Here's how the part is built. I have some questions about the finished solid (model axes, mm). A direction names the side the tool comes from. Give positions to 0.01 mm unless a question says otherwise; leave off trailing zeros. Write each loop counter-clockwise with the first axis right and the second up, starting at its lowest first coordinate (ties: lowest second). Pieces come first, ordered by that corner, then holes. Notation, with made-up numbers: (81, 73.5) - (94, 73.5) arc R20 ccw to (94, 111.5) - close; hole circle Ø3 at (38, -20.5). An arc over 180 degrees is marked (long way). One line per item, written item: value. Start each with the question number.
1) Imagine slicing it at B-B on x = 10. Write out the boundary of the cut face in (y, z), plus the area to 3 significant figures.
2) On a 3-axis mill with a long thin cutter (end or side, diameter ignored), from which of +Z, -Z, +X, -X, +Y, -Y can I reach the whole of each face in a straight line? I mean faces 3 (the flat face through (0, 15, 216)), 4 (the flat face through (22.7, -3, 215.9)), 5 (the flat face through (10, -2, 268)), 6 (the flat face through (10, -5, 274)). Say none if no direction works.
3) I'm going to push flat-ended pins straight in: P1, Ø2, axis at x = 0.5, y = 3.5, coming from the +Z side; P2, Ø0.6, axis at x = 13, y = -1, coming from the +Z side; P3, Ø1.2, axis at y = -5, z = 202, coming from the +X side; P4, Ø5, axis at y = 7, z = 186, coming from the +X side. Where does each tip first touch, or does it pass through?
4) Imagine slicing it at A-A on z = 215. Write out the boundary of the cut face in (x, y).
5) We'd pull the mould along Z, two halves only. Please class faces 1 (the flat face through (-2, -1, 216)), 2 (the cylindrical face through (10.35, -2.58, 158.44)): +Z half, -Z half, draft (parallel to the pull), parting line (faces both ways), or undercut.
6) Please list where these lines run through material, in increasing order: L1, parallel to Z at x = 10, y = -4; L2, parallel to Y at x = -1, z = 160; L3, parallel to Y at x = -4, z = 262. Write a range as [from, to].
7) Imagine slicing it at D-D on z = 252. Write out the boundary of the cut face in (x, y), plus the area to 3 significant figures.
from build123d import *

# Parameters (mm, degrees)
BOSS_EXTRUDE1_DEPTH            = 130
FILLET1_R                      = 1.5
SKETCH2_W                      = 130
SKETCH2_H                      = 3
BOSS_EXTRUDE2_DEPTH            = 10
SKETCH4_W                      = 13
SKETCH4_H                      = 130
BOSS_EXTRUDE3_DEPTH            = 4
SKETCH6_W                      = 3
SKETCH6_H                      = 130
BOSS_EXTRUDE4_DEPTH            = 10
SKETCH5_W                      = 130
SKETCH5_H                      = 13
BOSS_EXTRUDE5_DEPTH            = 4
CSK_FOR_M3_SFHCS1_D            = 3.2
CSK_FOR_M3_SFHCS1_CSINK_D      = 6.72
CSK_FOR_M3_SFHCS1_CSINK_ANGLE  = 90
CSK_FOR_M3_SFHCS2_D            = 3.2
CSK_FOR_M3_SFHCS2_CSINK_D      = 6.72
CSK_FOR_M3_SFHCS2_CSINK_ANGLE  = 90
SKETCH13_W                     = 12
SKETCH13_H                     = 24
CUT_EXTRUDE1_DEPTH             = 2
F_4_4_4_4_DIAMETER_HOLE1_D     = 4.4
F_4_4_4_4_DIAMETER_HOLE1_DEPTH = 3
SKETCH16_W                     = 24
SKETCH16_H                     = 12
CUT_EXTRUDE2_DEPTH             = 2
F_4_4_4_4_DIAMETER_HOLE2_D     = 4.4
F_4_4_4_4_DIAMETER_HOLE2_DEPTH = 3
F_4_4_4_4_DIAMETER_HOLE3_D     = 4.4
F_4_4_4_4_DIAMETER_HOLE4_D     = 4.4


with BuildPart() as part:
    # Sketch1 → Boss-Extrude1 (new body)
    with BuildSketch(Plane.XY.offset(280)):
        Polygon((-7, 4), (4, -7), (7, -7), (7, -3), (20, -3), (20, 0), (0, 0), (0, 20), (-3, 20), (-3, 7), (-7, 7), align=None)
    extrude(amount=-BOSS_EXTRUDE1_DEPTH)

    # Fillet1
    fillet1_edges = [part.edges().sort_by_distance(p)[0] for p in [
        (4, -7, 215),
        (-7, 4, 215),
    ]]
    fillet(fillet1_edges, radius=FILLET1_R)

    # Sketch2 → Boss-Extrude2 (add)
    with BuildSketch(Plane(origin=(20, 0, 0), x_dir=(0, 0, -1), z_dir=(1, 0, 0))):
        with Locations((-215, -1.5)):
            Rectangle(SKETCH2_W, SKETCH2_H)
    extrude(amount=BOSS_EXTRUDE2_DEPTH)

    # Sketch4 → Boss-Extrude3 (add)
    with BuildSketch(Plane.XZ.offset(3)):
        with Locations((13.5, 215)):
            Rectangle(SKETCH4_W, SKETCH4_H)
    extrude(amount=BOSS_EXTRUDE3_DEPTH)

    # Sketch6 → Boss-Extrude4 (add)
    with BuildSketch(Plane(origin=(0, 20, 0), x_dir=(1, 0, 0), z_dir=(0, 1, 0))):
        with Locations((-1.5, -215)):
            Rectangle(SKETCH6_W, SKETCH6_H)
    extrude(amount=BOSS_EXTRUDE4_DEPTH)

    # Sketch5 → Boss-Extrude5 (add)
    with BuildSketch(Plane.ZY.offset(3)):
        with Locations((215, 13.5)):
            Rectangle(SKETCH5_W, SKETCH5_H)
    extrude(amount=BOSS_EXTRUDE5_DEPTH)

    # CSK for M3 SFHCS1 (through all)
    with Locations(Plane.ZY.offset(7)):
        with Locations((160, 10)):
            CounterSinkHole(CSK_FOR_M3_SFHCS1_D / 2, CSK_FOR_M3_SFHCS1_CSINK_D / 2, counter_sink_angle=CSK_FOR_M3_SFHCS1_CSINK_ANGLE)

    # CSK for M3 SFHCS2 (through all)
    with Locations(Plane.XZ.offset(7)):
        with Locations((10, 160)):
            CounterSinkHole(CSK_FOR_M3_SFHCS2_D / 2, CSK_FOR_M3_SFHCS2_CSINK_D / 2, counter_sink_angle=CSK_FOR_M3_SFHCS2_CSINK_ANGLE)

    # Sketch13 → Cut-Extrude1 (cut)
    with BuildSketch(Plane(origin=(0, 0, 0), x_dir=(1, 0, 0), z_dir=(0, 1, 0))):
        with Locations((10, -268)):
            Rectangle(SKETCH13_W, SKETCH13_H)
    extrude(amount=-CUT_EXTRUDE1_DEPTH, mode=Mode.SUBTRACT)

    # Ø4.4 (4.4) Diameter Hole1
    with Locations(Plane(origin=(0, -2, 0), x_dir=(1, 0, 0), z_dir=(0, 1, 0))):
        with Locations((10, -262), (10, -274)):
            Hole(F_4_4_4_4_DIAMETER_HOLE1_D / 2, depth=F_4_4_4_4_DIAMETER_HOLE1_DEPTH)

    # Sketch16 → Cut-Extrude2 (cut)
    with BuildSketch(Plane(origin=(0, 0, 0), x_dir=(0, 0, -1), z_dir=(1, 0, 0))):
        with Locations((-268, 10)):
            Rectangle(SKETCH16_W, SKETCH16_H)
    extrude(amount=-CUT_EXTRUDE2_DEPTH, mode=Mode.SUBTRACT)

    # Ø4.4 (4.4) Diameter Hole2
    with Locations(Plane(origin=(-2, 0, 0), x_dir=(0, 0, -1), z_dir=(1, 0, 0))):
        with Locations((-262, 10), (-274, 10)):
            Hole(F_4_4_4_4_DIAMETER_HOLE2_D / 2, depth=F_4_4_4_4_DIAMETER_HOLE2_DEPTH)

    # Ø4.4 (4.4) Diameter Hole3 (through all)
    with Locations(Plane.ZY.offset(3)):
        with Locations((215, 25)):
            Hole(F_4_4_4_4_DIAMETER_HOLE3_D / 2)

    # Ø4.4 (4.4) Diameter Hole4 (through all)
    with Locations(Plane.XZ.offset(3)):
        with Locations((25, 215)):
            Hole(F_4_4_4_4_DIAMETER_HOLE4_D / 2)


solid = part.part
Numbers:
1. outline: (-7, 150) - (0, 150) - (0, 158.4) - (-5.24, 158.4) - (-7, 156.64) - close; (-7, 163.36) - (-5.24, 161.6) - (0, 161.6) - (0, 256) - (-2, 256) - (-2, 259.8) - (-5, 259.8) - (-5, 264.2) - (-2, 264.2) - (-2, 271.8) - (-5, 271.8) - (-5, 276.2) - (-2, 276.2) - (-2, 280) - (-7, 280) - close
1. area: 810 mm^2
2. face 3: +Z, -Z, +X, +Y
2. face 4: +Z, -Z, +X, -Y
2. face 5: +Z, +Y
2. face 6: +Y
3. P1: z = 280
3. P2: z = 256
3. P3: x = 20
3. P4: x = 0
4. outline: (-7, 4.62) arc R1.5 ccw to (-6.56, 3.56) - (3.56, -6.56) arc R1.5 ccw to (4.62, -7) - (20, -7) - (20, -3) - (22.8, -3) - (22.8, 0) - (0, 0) - (0, 22.8) - (-3, 22.8) - (-3, 20) - (-7, 20) - close; (-3, 27.2) - (0, 27.2) - (0, 30) - (-3, 30) - close; (27.2, -3) - (30, -3) - (30, 0) - (27.2, 0) - close
5. face 1: draft
5. face 2: undercut
6. L1: [150, 158.4], [161.6, 259.8], [264.2, 271.8], [276.2, 280]
6. L2: [-2, 8.4], [11.6, 30]
6. L3: [1, 7.8], [12.2, 20]
7. outline: (-7, 4.62) arc R1.5 ccw to (-6.56, 3.56) - (3.56, -6.56) arc R1.5 ccw to (4.62, -7) - (20, -7) - (20, -3) - (30, -3) - (30, 0) - (0, 0) - (0, 30) - (-3, 30) - (-3, 20) - (-7, 20) - close
7. area: 328 mm^2
